Input: part model. Units: mm. Frame: model coordinates. Face numbers are marked on the shaded views. A direction names the side the tool comes from. Give positions to 0.01 mm unless a question says otherwise; leave off trailing zeros. Write each loop counter-clockwise with the first axis right and the second up, starting at its lowest first coordinate (ties: lowest second). Pieces come first, ordered by that corner, then holes.
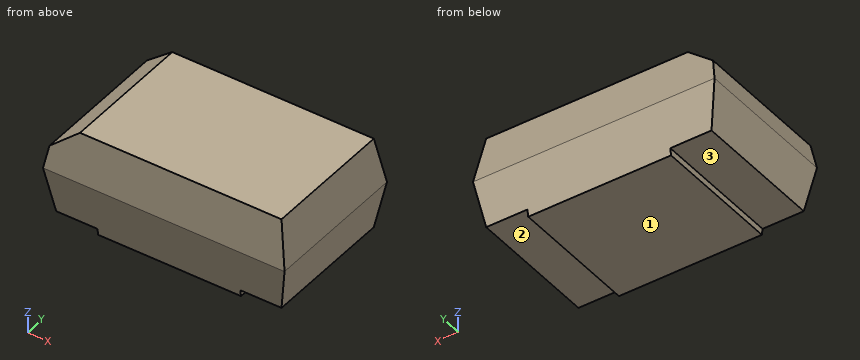
```python
from build123d import *

# Parameters (mm, degrees)
PAD002_DEPTH    = 2.15
POCKET004_DEPTH = 10
POCKET005_DEPTH = 12.5
CHAMFER001_SIZE = 0.7


with BuildPart() as part:
    # Sketch011 → Pad002 (new body, symmetric)
    with BuildSketch(Plane.XZ):
        Polygon((-3.311958576, 2.9), (3.311958576, 2.9), (3.55, 1.55), (3.311958576, 0.2), (2.1, 0.2), (2.1, 0), (-2.1, 0), (-2.1, 0.2), (-3.311958576, 0.2), (-3.55, 1.55), align=None)
    extrude(amount=PAD002_DEPTH, both=True)

    # Sketch012 → Pocket004 (cut, symmetric)
    with BuildSketch(Plane(origin=(2.1, 0, 0), x_dir=(0, 0, 1), z_dir=(1, 0, 0))):
        Polygon((2.9220926693, 2.229851), (3.3067026402, 1.8717656945), (1.045841, 2.229851), align=None)
        Polygon((3.3067026402, -1.8717656945), (2.9220926693, -2.229851), (1.045841, -2.229851), align=None)
    extrude(amount=POCKET004_DEPTH, both=True, mode=Mode.SUBTRACT)

    # Sketch013 → Pocket005 (cut, symmetric)
    with BuildSketch(Plane(origin=(2.1, 0, 0), x_dir=(0, 0, 1), z_dir=(1, 0, 0))):
        Polygon((2.1937543082, 2.2519614985), (-0.4776096389, 2.2519614985), (-0.6097972306, 1.8079225571), align=None)
        Polygon((2.1937543082, -2.2519614985), (-0.4776096389, -2.2519614985), (-0.6097972306, -1.8079225571), align=None)
    extrude(amount=POCKET005_DEPTH, both=True, mode=Mode.SUBTRACT)

    # Chamfer001
    chamfer001_edges = [part.edges().sort_by_distance(p)[0] for p in [
        (-3.311959, 0, 2.9),
    ]]
    chamfer(chamfer001_edges, length=CHAMFER001_SIZE)


solid = part.part
```
Item 1: Section A-A (y = 0.8). Return loops of the section in (x, z).
Item 2: Set-up query: the marked faces 1, 2 and 3. Return all of +Z, -Z, +X, -X, +Y, -Y with unobstructed straight access to the full face (end or side cutting, diameter ignored); none if empty.
Item 3: Ray query, line 1 (Z direction, x = -2.25, y = 0.9); line 2 (X direction, y = 0.05, z = 1.75); line 3 (X direction, y = 1.9, z = 0.3). Return the intervals inside material, ascending.
Item 4: Section D-D (z = 2.6). Return loops of the section in (x, y).
Item 5: Pin query (flat end, axial travel): pin 1 (1.3 mm diameter, centred on x = 3, y = -0.5, fed in from -Z). Return the tip coordinate at first contact, or that it passes through.
Solved:
1. outline: (-3.55, 1.55) - (-3.31, 0.2) - (-2.1, 0.2) - (-2.1, 0) - (2.1, 0) - (2.1, 0.2) - (3.31, 0.2) - (3.55, 1.55) - (3.31, 2.9) - (-2.61, 2.9) - (-3.43, 2.21) - close
2. face 1: -Z, +X, -X, +Y, -Y
2. face 2: -Z, +X, +Y, -Y
2. face 3: -Z, -X, +Y, -Y
3. line 1: z = 0.2 to 2.9
3. line 2: x = -3.51 to 3.51
3. line 3: x = -3.33 to 3.33
4. outline: (-2.97, -1.98) - (3.36, -1.98) - (3.36, 1.98) - (-2.97, 1.98) - close
5. pin 1: stops at z = 0.2
